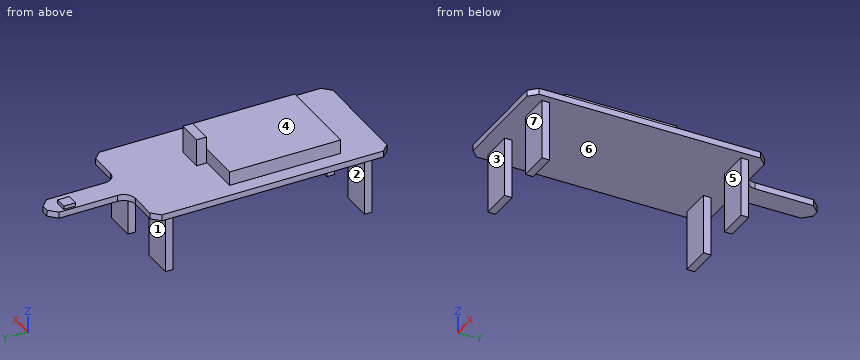
from build123d import *

# Parameters (mm, degrees)
F1_DEPTH = 1.6
F2_W     = 22
F2_H     = 28.6
F3_DEPTH = 3.6
F2_W_2   = 6.5
F2_H_2   = 2.5
F4_DEPTH = 7
F2_W_3   = 3
F2_H_3   = 3
F5_DEPTH = 0.9
F6_W     = 8
F6_H     = 2
F7_DEPTH = 15.4
F8_R     = 3
F9_SIZE  = 2


with BuildPart() as f1:
    # F0 (on Top) → F1 (new body)
    with BuildSketch(Plane.XY):
        Polygon((-3, 30.5), (-15, 30.5), (-15, -30.5), (15, -30.5), (15, 30.5), (3, 30.5), (3, 50.5), (-3, 50.5), align=None)
    extrude(amount=F1_DEPTH)

    # F2 (on face) → F3 (join)
    with BuildSketch(Plane.XY.offset(1.6)):
        with Locations((-0.3, -5.2)):
            Rectangle(F2_W, F2_H)
    extrude(amount=F3_DEPTH)

    # F2 (on face) → F4 (join)
    with BuildSketch(Plane.XY.offset(1.6)):
        with Locations((2.75, 10.55)):
            Rectangle(F2_W_2, F2_H_2)
    extrude(amount=F4_DEPTH)

    # F2 (on face) → F5 (join)
    with BuildSketch(Plane.XY.offset(1.6)):
        with Locations((-1, 45.5)):
            Rectangle(F2_W_3, F2_H_3)
    extrude(amount=F5_DEPTH)

    # F6 (on face) → F7 (join)
    with BuildSketch(Plane(origin=(0, 0, 0), x_dir=(1, 0, 0), z_dir=(0, 0, -1))):
        with Locations((-9, 25.7)):
            Rectangle(F6_W, F6_H)
        with Locations((9, 25.7)):
            Rectangle(F6_W, F6_H)
        with Locations((-9, -25.5)):
            Rectangle(F6_W, F6_H)
        with Locations((9, -25.5)):
            Rectangle(F6_W, F6_H)
    extrude(amount=F7_DEPTH)

    # F8
    f8_edges = [f1.edges().sort_by_distance(p)[0] for p in [
        (-3, 30.5, 0.8),
        (3, 30.5, 0.8),
    ]]
    fillet(f8_edges, radius=F8_R)

    # F9
    f9_edges = [f1.edges().sort_by_distance(p)[0] for p in [
        (-15, 30.5, 0.8),
        (-15, -30.5, 0.8),
        (15, -30.5, 0.8),
        (15, 30.5, 0.8),
        (3, 50.5, 0.8),
        (-3, 50.5, 0.8),
    ]]
    chamfer(f9_edges, length=F9_SIZE)


solid = f1.part
Design review of the part built by this model. Coordinates are the model's own, in mm. Face numbers are marked on the shaded views. A direction names the side the tool comes from. Coordinates: 2 decimals unless noted, no trailing zeros. Order: outer loops, then holes, each group sorted by start corner. A loop starts at its lowest first (then second) coordinate and runs counter-clockwise, first axis right, second up. Notation, with made-up numbers: M -27.5,51.25 L -3.5,51.25 A37 cw -3.5,90.25 Z; hole C 76,52 d6. An arc over 180 degrees is marked long. Use a Markdown table: item, result.
(1) Draft analysis for pull direction Y (two halves, no side actions). For the marked faces 4, 5, 6 and 7, state which applies: released by +Y, released by -Y, zero draft, split by the parting line, or undercut.
Worked answers:
| item | result |
|---|---|
| face 4 | zero draft |
| face 5 | undercut |
| face 6 | undercut |
| face 7 | released by -Y |
(2) Add section C-C (x = 12). Give the boundary of the cut face in (y, z).
Worked answers:
| item | result |
|---|---|
| outline | M -30.5,0 L -26.7,0 L -26.7,-15.4 L -24.7,-15.4 L -24.7,0 L 24.5,0 L 24.5,-15.4 L 26.5,-15.4 L 26.5,0 L 30.5,0 L 30.5,1.6 L -30.5,1.6 Z |
(3) Wall thickness on probe 1 along Y at (x, z) = (11.5, -8); probe 2 along X at (y, z) = (-26.5, -9); probe 3 along Z at (x, y) = (-8.5, 7.5): over which ranges is each line inside the solid? List them lowest first.
Worked answers:
| item | result |
|---|---|
| probe 1 | y = -26.7 to -24.7, 24.5 to 26.5 |
| probe 2 | x = -13 to -5, 5 to 13 |
| probe 3 | z = 0 to 5.2 |
(4) Add section B-B (z = -6.5). Give the boundary of the cut face in (x, y), then the cut area to 3 significant figures.
Worked answers:
| item | result |
|---|---|
| outline | M -13,-26.7 L -5,-26.7 L -5,-24.7 L -13,-24.7 Z; M -13,24.5 L -5,24.5 L -5,26.5 L -13,26.5 Z; M 5,-26.7 L 13,-26.7 L 13,-24.7 L 5,-24.7 Z; M 5,24.5 L 13,24.5 L 13,26.5 L 5,26.5 Z |
| area | 64.0 mm2 |
(5) Add section A-A (z = 3.5). Give the boundary of the cut face in (x, y).
Worked answers:
| item | result |
|---|---|
| outline | M -11.3,-19.5 L 10.7,-19.5 L 10.7,9.1 L -11.3,9.1 Z; M -0.5,9.3 L 6,9.3 L 6,11.8 L -0.5,11.8 Z |
(6) For P1, Ø1, axis at x = -1, z = 2, coming from the +Y side; P2, Ø2.5, axis at x = 8, z = -10.5, coming from the -Y side; P3, Ø3, axis at y = -11.5, z = 4, coming from the -X side; P4, Ø2, axis at y = -26, z = -5, coming from the -X side, all flat-tipped, find the tip position at first contact; note any pin that passes through.
Worked answers:
| item | result |
|---|---|
| P1 | stops at y = 50.5 |
| P2 | stops at y = -26.7 |
| P3 | stops at x = -11.3 |
| P4 | stops at x = -13 |
(7) For the marked faces 1, 2 and 3, list the 3-axis set-ups (+Z, -Z, +X, -X, +Y, -Y) from which the entire face can be reached by the end or side of a thin tool; tool diameter is ignored.
Worked answers:
| item | result |
|---|---|
| face 1 | -Z, +X, -X, +Y |
| face 2 | -Z, +X, -X |
| face 3 | -Z, +X, -X, -Y |
(8) Add section D-D (y = -13). Give the boundary of the cut face in (x, z), then the cut area to 3 significant figures.
Worked answers:
| item | result |
|---|---|
| outline | M -15,0 L 15,0 L 15,1.6 L 10.7,1.6 L 10.7,5.2 L -11.3,5.2 L -11.3,1.6 L -15,1.6 Z |
| area | 127 mm2 |
